```python
from build123d import *

# Parameters (mm, degrees)
F0_W     = 1270
F0_H     = 1955.8
F1_DEPTH = 203.2
F2_W     = 1270
F2_H     = 1524
F3_DEPTH = 12.7
F4_W     = 558.8
F4_H     = 330.2
F5_DEPTH = 76.2
F6_R     = 25.4
F7_R     = 25.4


with BuildPart() as f1:
    # F0 (on Top) → F1 (new body)
    with BuildSketch(Plane.XY):
        with Locations((-7.088182494, 100.0628365508)):
            Rectangle(F0_W, F0_H)
    extrude(amount=F1_DEPTH)

    # F2 (on face) → F3 (join)
    with BuildSketch(Plane.XY.offset(203.2)):
        with Locations((-7.088182494, -115.8371634492)):
            Rectangle(F2_W, F2_H)
    extrude(amount=F3_DEPTH)

    # F4 (on face) → F5 (join)
    with BuildSketch(Plane.XY.offset(203.2)):
        with Locations((-311.888182494, 862.0628365508)):
            Rectangle(F4_W, F4_H)
        with Locations((297.711817506, 862.0628365508)):
            Rectangle(F4_W, F4_H)
    extrude(amount=F5_DEPTH)

    # F6
    f6_edges = [f1.edges().sort_by_distance(p)[0] for p in [
        (-32.488182, 1027.162837, 241.3),
        (-32.488182, 696.962837, 241.3),
        (18.311818, 696.962837, 241.3),
        (18.311818, 1027.162837, 241.3),
        (577.111818, 696.962837, 241.3),
        (577.111818, 1027.162837, 241.3),
        (-591.288182, 1027.162837, 241.3),
        (-591.288182, 696.962837, 241.3),
    ]]
    fillet(f6_edges, radius=F6_R)

    # F7
    f7_edges = [f1.edges().sort_by_distance(p)[0] for p in [
        (-311.888182, 1027.162837, 279.4),
        (-32.488182, 862.062837, 279.4),
        (-39.92767, 1019.723349, 279.4),
        (-39.92767, 704.402324, 279.4),
        (-311.888182, 696.962837, 279.4),
        (-583.848695, 704.402324, 279.4),
        (-591.288182, 862.062837, 279.4),
        (-583.848695, 1019.723349, 279.4),
        (18.311818, 862.062837, 279.4),
        (25.751305, 1019.723349, 279.4),
        (297.711818, 1027.162837, 279.4),
        (569.67233, 1019.723349, 279.4),
        (577.111818, 862.062837, 279.4),
        (569.67233, 704.402324, 279.4),
        (297.711818, 696.962837, 279.4),
        (25.751305, 704.402324, 279.4),
    ]]
    fillet(f7_edges, radius=F7_R)


solid = f1.part
```
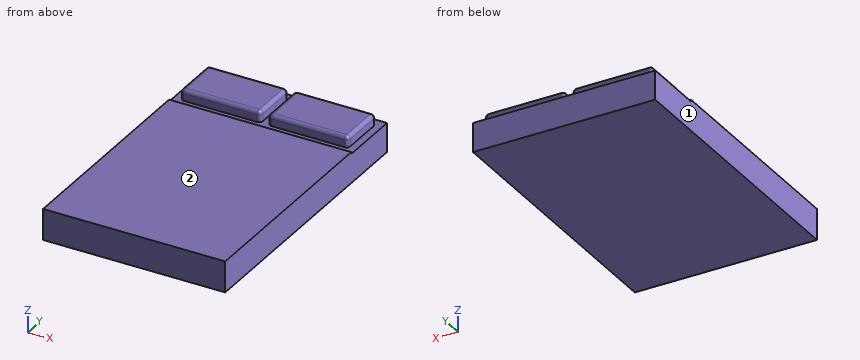
Model file for the job. Use its own axes, mm. Face numbers are marked on the shaded views. A direction names the side the tool comes from. Give positions to 0.01 mm unless a question says otherwise; leave off trailing zeros. Write each loop counter-clockwise with the first axis right and the second up, starting at its lowest first coordinate (ties: lowest second). Pieces come first, ordered by that corner, then holes. Notation, with made-up numbers: (78.5, -23) - (123.5, -23) arc R30 cw to (123.5, -1) - close; hole circle Ø10 at (-32, 42.25). An arc over 180 degrees is marked (long way). One line per question, with ' | ' between items. Start each with the question number.
(1) Slice it at B-B on x = -392. Write the cut outline in (y, z), plus the area to 3 significant figures.
(2) Wall check: line 1 along Z through (x, y) = (555.5, -776.5); line 2 along Y through (x, z) = (180.5, 230); line 3 along Y through (x, z) = (468, 255). Give the ranges that are in metal, low to high. Write a range as from..to.
(3) Pin check, flat tips, straight feed: P1, Ø3, axis at x = -136.5, y = -172, coming from the -Z side; P2, Ø12, axis at x = -213, y = 307, coming from the +Z side; P3, Ø15, axis at x = 252.5, z = 237, coming from the -Y side. Stop position of each tip, or through.
(4) Slice it at A-A on y = 744.5. Write the cut outline in (x, z), plus the area to 3 significant figures.
(5) Slice it at C-C on y = 118.5. Write the cut outline in (x, z), plus the area to 3 significant figures.
(6) 3-axis set-ups, long thin cutter, end or side, ignore diameter. For the marked faces 1 and 2: which of +Z, -Z, +X, -X, +Y, -Y reach the whole face in a straight line?
Results below:
1) outline: (-877.84, 0) - (1077.96, 0) - (1077.96, 203.2) - (1027.16, 203.2) - (1027.16, 254) arc R25.4 ccw to (1001.76, 279.4) - (722.36, 279.4) arc R25.4 ccw to (696.96, 254) - (696.96, 203.2) - (646.16, 203.2) - (646.16, 215.9) - (-877.84, 215.9) - close | area: 442,000 mm^2
2) line 1: 0..215.9 | line 2: 696.96..1027.16 | line 3: 696.98..1027.14
3) P1: z = 0 | P2: z = 215.9 | P3: y = 696.96
4) outline: (-642.09, 0) - (627.91, 0) - (627.91, 203.2) - (577.11, 203.2) - (577.11, 254) arc R25.4 ccw to (551.71, 279.4) - (43.71, 279.4) arc R25.4 ccw to (18.31, 254) - (18.31, 203.2) - (-32.49, 203.2) - (-32.49, 254) arc R25.4 ccw to (-57.89, 279.4) - (-565.89, 279.4) arc R25.4 ccw to (-591.29, 254) - (-591.29, 203.2) - (-642.09, 203.2) - close | area: 343,000 mm^2
5) outline: (-642.09, 0) - (627.91, 0) - (627.91, 215.9) - (-642.09, 215.9) - close | area: 274,000 mm^2
6) face 1: +Z, -Z, -X, +Y, -Y | face 2: +Z, +X, -X, -Y
